from build123d import *

# Parameters (mm, degrees)
SKETCH3_R       = 2.55
EXTRUDE2_DEPTH  = 4.7
EXTRUDE3_DEPTH  = 5.7
SKETCH13_W      = 0.45
SKETCH13_H      = 0.45
EXTRUDE8_DEPTH  = 0.1
SKETCH12_W      = 0.45
SKETCH12_H      = 0.45
EXTRUDE9_DEPTH  = 0.1
SKETCH11_W      = 0.45
SKETCH11_H      = 0.45
EXTRUDE10_DEPTH = 1.598630162
SKETCH32_W      = 0.45
SKETCH32_H      = 0.45
REVOLVE4_ANGLE  = 45
SKETCH34_W      = 0.45
SKETCH34_H      = 0.45
EXTRUDE12_DEPTH = 1.61
SKETCH36_W      = 0.45
SKETCH36_H      = 0.45
REVOLVE5_ANGLE  = 45
SKETCH37_W      = 0.45
SKETCH37_H      = 0.45
EXTRUDE13_DEPTH = 3.04
SKETCH38_W      = 0.45
SKETCH38_H      = 0.45
REVOLVE6_ANGLE  = 45
SKETCH39_W      = 0.45
SKETCH39_H      = 0.45
EXTRUDE14_DEPTH = 1.61
SKETCH40_W      = 0.45
SKETCH40_H      = 0.45
REVOLVE7_ANGLE  = 45
SKETCH41_W      = 0.45
SKETCH41_H      = 0.45
EXTRUDE15_DEPTH = 3.04
SKETCH42_W      = 0.45
SKETCH42_H      = 0.45
EXTRUDE16_DEPTH = 3


with BuildPart() as part:
    # Sketch3 → Extrude2 (new body)
    with BuildSketch(Plane(origin=(0, 0, 0), x_dir=(1, 0, 0), z_dir=(0, 1, 0))):
        Circle(SKETCH3_R)
    extrude(amount=EXTRUDE2_DEPTH)

    # Sketch3_3 → Extrude3 (cut, through all)
    with BuildSketch(Plane(origin=(0, 0, 0), x_dir=(1, 0, 0), z_dir=(0, 1, 0))):
        Polygon((-24.311295597, 1.55), (-2.024845673, 1.55), (2.024845673, 1.55), (24.311295597, 1.55), (24.311295597, 46.122899848), (-24.311295597, 46.122899848), align=None)
    extrude(amount=EXTRUDE3_DEPTH, mode=Mode.SUBTRACT)

    # Sketch13 → Extrude8 (add)
    with BuildSketch(Plane.XZ):
        with Locations((1.27, 0)):
            Rectangle(SKETCH13_W, SKETCH13_H)
    extrude(amount=EXTRUDE8_DEPTH)

    # Sketch12 → Extrude9 (add)
    with BuildSketch(Plane.XZ):
        with Locations((-1.27, 0)):
            Rectangle(SKETCH12_W, SKETCH12_H)
    extrude(amount=EXTRUDE9_DEPTH)

    # Sketch11 → Extrude10 (add)
    with BuildSketch(Plane.XZ):
        Rectangle(SKETCH11_W, SKETCH11_H)
    extrude(amount=EXTRUDE10_DEPTH)

    # Sketch32 → Revolve4 (revolve)
    with BuildSketch(Plane.XZ.offset(0.1)):
        with Locations((-1.27, 0)):
            Rectangle(SKETCH32_W, SKETCH32_H)
    revolve(axis=Axis((-1.495, -0.1, 0.225), (0, 0, -1)), revolution_arc=REVOLVE4_ANGLE)

    # Sketch34 → Extrude12 (add)
    with BuildSketch(Plane(origin=(-0.7975, -0.7975, 0), x_dir=(0, 0, 1), z_dir=(-0.707106781, -0.707106781, 0))):
        with Locations((0, 0.76141396)):
            Rectangle(SKETCH34_W, SKETCH34_H)
    extrude(amount=EXTRUDE12_DEPTH)

    # Sketch36 → Revolve5 (revolve)
    with BuildSketch(Plane(origin=(-1.935941918, -1.935941918, 0), x_dir=(0, 0, 1), z_dir=(-0.707106781, -0.707106781, 0))):
        with Locations((0, 0.76141396)):
            Rectangle(SKETCH36_W, SKETCH36_H)
    revolve(axis=Axis((-2.315243866, -1.556639969, -0.225), (0, 0, 1)), revolution_arc=REVOLVE5_ANGLE)

    # Sketch37 → Extrude13 (add)
    with BuildSketch(Plane.XZ.offset(1.556639969)):
        with Locations((-2.540243866, 0)):
            Rectangle(SKETCH37_W, SKETCH37_H)
    extrude(amount=EXTRUDE13_DEPTH)

    # Sketch38 → Revolve6 (revolve)
    with BuildSketch(Plane.XZ.offset(0.1)):
        with Locations((1.27, 0)):
            Rectangle(SKETCH38_W, SKETCH38_H)
    revolve(axis=Axis((1.495, -0.1, 0.225), (0, 0, 1)), revolution_arc=REVOLVE6_ANGLE)

    # Sketch39 → Extrude14 (add)
    with BuildSketch(Plane(origin=(0.7975, -0.7975, 0), x_dir=(0, 0, -1), z_dir=(0.707106781, -0.707106781, 0))):
        with Locations((0, 0.76141396)):
            Rectangle(SKETCH39_W, SKETCH39_H)
    extrude(amount=EXTRUDE14_DEPTH)

    # Sketch40 → Revolve7 (revolve)
    with BuildSketch(Plane(origin=(1.935941918, -1.935941918, 0), x_dir=(0, 0, -1), z_dir=(0.707106781, -0.707106781, 0))):
        with Locations((0, 0.76141396)):
            Rectangle(SKETCH40_W, SKETCH40_H)
    revolve(axis=Axis((2.315243866, -1.556639969, 0.225), (0, 0, -1)), revolution_arc=REVOLVE7_ANGLE)

    # Sketch41 → Extrude15 (add)
    with BuildSketch(Plane.XZ.offset(1.556639969)):
        with Locations((2.540243866, 0)):
            Rectangle(SKETCH41_W, SKETCH41_H)
    extrude(amount=EXTRUDE15_DEPTH)

    # Sketch42 → Extrude16 (add)
    with BuildSketch(Plane.XZ.offset(1.598630162)):
        Rectangle(SKETCH42_W, SKETCH42_H)
    extrude(amount=EXTRUDE16_DEPTH)


solid = part.part
Part model, mm, in its own coordinate system. A direction names the side the tool comes from. Coordinates: 2 decimals unless noted, no trailing zeros. Order: outer loops, then holes, each group sorted by start corner. A loop starts at its lowest first (then second) coordinate and runs counter-clockwise, first axis right, second up. Notation, with made-up numbers: M -39,-11 L 12,-11 A27 cw 12,28 Z; hole C -37.75,-17.5 d6. An arc over 180 degrees is marked long. One line per question, with ' | ' between items.
Q1. 3-axis set-ups, long thin cutter, end or side, ignore diameter. For faces 1 (the face through (1.74, -0.98, 0)), 2 (the face through (2.056, -0.661, 0.003)), 3 (the face through (2.5, -2.3, 0.225)), 4 (the face through (2.5, -2.3, -0.225)): which of +Z, -Z, +X, -X, +Y, -Y reach the whole face in a straight line?
A:
face 1: +Z, -Z, -Y | face 2: +Z, -Z, +X | face 3: +Z, +X, -X, -Y | face 4: -Z, +X, -X, -Y
Q2. Slice it at A-A (y = -2). Give the cut face in (x, z) (3 decimals).
A:
outline: M -2.765,-0.225 L -2.315,-0.225 L -2.315,0.225 L -2.765,0.225 Z; M -0.225,-0.225 L 0.225,-0.225 L 0.225,0.225 L -0.225,0.225 Z; M 2.315,-0.225 L 2.765,-0.225 L 2.765,0.225 L 2.315,0.225 Z
Q3. Slice it at C-C (z = 0). Give the cut face in (x, y) (3 decimals).
A:
outline: M -2.765,-4.597 L -2.315,-4.597 L -2.315,-1.557 L -1.177,-0.418 A0.45 ccw -1.045,-0.1 L -1.045,0 L -0.225,0 L -0.225,-4.599 L 0.225,-4.599 L 0.225,0 L 1.045,0 L 1.045,-0.1 A0.45 ccw 1.177,-0.418 L 2.315,-1.557 L 2.315,-4.597 L 2.765,-4.597 L 2.765,-1.557 A0.45 ccw 2.633,-1.238 L 1.495,-0.1 L 1.495,0 L 2.55,0 L 2.55,4.7 L -2.55,4.7 L -2.55,0 L -1.495,0 L -1.495,-0.1 L -2.633,-1.238 A0.45 ccw -2.765,-1.557 Z
Q4. Two-plate mould, pull along Y, no slides. Class faces 5 (the face through (-2.056, -0.661, -0.003)), 6 (the face through (-0.08, 2.32, 2.55)), 7 (the face through (-1.74, -0.98, 0)), 8 (the face through (0, 4.7, 0)): +Y half, -Y half, draft (parallel to the pull), parting line (faces both ways), or undercut.
A:
face 5: undercut | face 6: draft | face 7: -Y half | face 8: +Y half
Q5. Slice it at D-D (y = 2). Give the cut face in (x, z).
A:
outline: M -2.02,-1.55 L 2.02,-1.55 A2.55 ccw long Z
Q6. Slice it at B-B (x = 0). Give the cut face in (y, z) (3 decimals).
A:
outline: M -4.599,-0.225 L 0,-0.225 L 0,-1.55 L 4.7,-1.55 L 4.7,2.55 L 0,2.55 L 0,0.225 L -4.599,0.225 Z
Q7. Pin check, flat tips, straight feed: P1, Ø0.5, axis at x = 2, y = -1.5, coming from the -Z side (3 decimals); P2, Ø1.2, axis at x = -0.5, z = 0, coming from the -Y side; P3, Ø0.5, axis at x = -2, y = -1.5, coming from the +Z side (3 decimals); P4, Ø2, axis at y = 1, z = -0.5, coming from the -X side. Stop position of each tip, or through.
A:
P1: stops at z = -0.225 | P2: stops at y = -4.6 | P3: stops at z = 0.225 | P4: stops at x = -2.55
Q8. Drill centre lines: line 1 (X direction, y = -0.75, z = 0.1) (3 decimals); line 2 (Y direction, x = -1.25, z = -0.4); line 3 (Z direction, x = -2.5, y = -4) (3 decimals). Where is each one in solid material? Low to high.
A:
line 1: x = -2.145 to -1.509, -0.225 to 0.225, 1.509 to 2.145 | line 2: y = 0 to 4.7 | line 3: z = -0.225 to 0.225
